```python
from build123d import *

# Parameters (mm, degrees)
F_0165_CONE_ROTATE_ANGLE    = 90
F_0166_CYLINDER_SKETCH_R    = 1.2
F_0166_CYLINDER_DEPTH       = 10.05
F_0167_CONE_ROTATE_ANGLE    = 90
F_0172_EXTRUDE_DEPTH        = 1.033
F_0172_EXTRUDE_ROTATE_ANGLE = 120


with BuildPart() as part:
    # 0165_cone_Sketch → 0165_cone (revolve)
    with BuildSketch(Plane.XY, mode=Mode.PRIVATE) as f_0165_cone_sk:
        Polygon((0, 0), (1.2, 0), (2.75, 1.65), (0, 1.65), align=None)
    revolve(f_0165_cone_sk.sketch.rotate(Axis((0, -100, 0), (0, 1, 0)), 90), axis=Axis((0, -100, 0), (0, 1, 0)))


with BuildPart() as part_1:
    # 0165_cone_Rotate: moved
    add(part.part.rotate(Axis((0, 0, 0), (1, 0, 0)), F_0165_CONE_ROTATE_ANGLE))


with BuildPart() as part_2:
    # 0165_cone_Translate: moved
    add(part_1.part.moved(Location((0, 0, -1.65))))


with BuildPart() as body_2:
    # 0166_cylinder_Sketch → 0166_cylinder (new body)
    with BuildSketch(Plane.XY):
        Circle(F_0166_CYLINDER_SKETCH_R)
    extrude(amount=F_0166_CYLINDER_DEPTH)


with BuildPart() as body_2_1:
    # 0166_cylinder_Translate: moved
    add(body_2.part.moved(Location((0, 0, -11.7))))


with BuildPart() as body_3:
    # 0167_cone_Sketch → 0167_cone (revolve)
    with BuildSketch(Plane.XY, mode=Mode.PRIVATE) as f_0167_cone_sk:
        Polygon((0, 0), (1.2, 0), (0.9, 0.3), (0, 0.3), align=None)
    revolve(f_0167_cone_sk.sketch.rotate(Axis((0, -100, 0), (0, 1, 0)), 90), axis=Axis((0, -100, 0), (0, 1, 0)))


with BuildPart() as body_3_1:
    # 0167_cone_Rotate: moved
    add(body_3.part.rotate(Axis((0, 0, 0), (1, 0, 0)), F_0167_CONE_ROTATE_ANGLE))


with BuildPart() as body_3_2:
    # 0167_cone_Translate: moved
    add(body_3_1.part.moved(Location((0, 0, -12))))


with BuildPart() as body_2_2:
    add(body_2_1.part)

    # 0169_add: union body 3
    add(body_3_2.part)


with BuildPart() as part_3:
    add(part_2.part)

    # 0171_add: union body 2
    add(body_2_2.part)


with BuildPart() as body_2_2_1:
    # 0172_extrude_Sketch → 0172_extrude (new body)
    with BuildSketch(Plane.XY):
        Polygon((0, 0), (1.154700538, 0), (1.732050808, 1), (1.154700538, 2), (0, 2), (-0.577350269, 1), align=None)
    extrude(amount=F_0172_EXTRUDE_DEPTH)


with BuildPart() as body_2_2_2:
    # 0172_extrude_Rotate: moved
    add(body_2_2_1.part.rotate(Axis((0, 0, 0), (0, 0, 1)), F_0172_EXTRUDE_ROTATE_ANGLE))


with BuildPart() as body_2_2_3:
    # 0172_extrude_Translate: moved
    add(body_2_2_2.part.moved(Location((1.154700538, 0, -1.023))))


with BuildPart() as part_4:
    add(part_3.part)

    # 0174_sub: cut body 2 2
    add(body_2_2_3.part, mode=Mode.SUBTRACT)


solid = part_4.part
```
Check sheet for the modelled part. Datum: model origin and axes. Units: mm. A direction names the side the tool comes from. Give positions to 0.01 mm unless a question says otherwise; leave off trailing zeros. Order: outer loops, then holes, each group sorted by start corner. A loop starts at its lowest first (then second) coordinate and runs counter-clockwise, first axis right, second up. Notation, with made-up numbers: M 24.5,80 L 59.5,80 A11 cw 59.5,94 Z; hole C -25,73 d8. An arc over 180 degrees is marked long. Answer in a Markdown table with one row per item.
1) Cross-section at A-A, the plane x = 0. Enter the section's corners in (y, z).
Filled sheet:
| item | result |
|---|---|
| outline | M -2.75,0 L -1.2,-1.65 L -1.2,-11.7 L -0.9,-11.7 L -1.2,-12 L 1.2,-12 L 0.9,-11.7 L 1.2,-11.7 L 1.2,-1.65 L 2.75,0 L 1,0 L 1,-1.02 L -1,-1.02 L -1,0 Z |
2) Cross-section at B-B, the plane z = -10.75. Enter the section's corners in (x, y), plus the area to 3 significant figures.
Filled sheet:
| item | result |
|---|---|
| outline | C 0,0 d2.4 |
| area | 4.52 mm2 |
3) Access from +Z, -Z, +X, -X, +Y, -Y to the whole of each face (thin tool, end or side, straight path). Record for faces 1 (the flat face through (0, 0, -12)), 2 (the cylindrical face through (0.65, 1.01, -6.75)), 3 (the flat face through (-0.86, 0.51, -0.52)).
Filled sheet:
| item | result |
|---|---|
| face 1 | -Z, +X, -X, +Y, -Y |
| face 2 | -Z |
| face 3 | +Z |
4) Thickness scan on L1, parallel to Z at x = 0, y = 0.6; L2, parallel to Z at x = -1.8, y = 1.55; L3, parallel to X at y = 0.25, z = -6.25. Record the ranges inside material, lowest first. Write a range as [from, to].
Filled sheet:
| item | result |
|---|---|
| L1 | z = [-12, -1.02] |
| L2 | z = [-0.4, 0] |
| L3 | x = [-1.17, 1.17] |
5) Gauge pin test, flat ends, axial feed: P1, Ø0.5, axis at x = 0, z = -0.5, coming from the -Y side; P2, Ø2, axis at x = 1, z = -3, coming from the -Y side; P3, Ø1.5, axis at x = 0, z = -5, coming from the +Y side. Record the tip position at first contact, or that the pin passes through.
Filled sheet:
| item | result |
|---|---|
| P1 | stops at y = -2.52 |
| P2 | stops at y = -1.2 |
| P3 | stops at y = 1.2 |
